Here's how the part is built. I have some questions about the finished solid (model axes, mm). Coordinates: 2 decimals unless noted, no trailing zeros. Write each loop counter-clockwise with the first axis right and the second up, starting at its lowest first coordinate (ties: lowest second). Pieces come first, ordered by that corner, then holes.
Item 1: I want a section at A-A (x = 0). Please give me the cut outline in (y, z), and give its area (3 significant figures).
Item 2: I want a section at D-D (z = 22). Please give me the cut outline in (x, y), and give its area (3 significant figures).
Item 3: I'm going to push flat-ended pins straight in: P1, Ø14.5, axis at x = 0, y = 0, coming from the -Z side; P2, Ø2, axis at y = -10, z = 10.5, coming from the -X side; P3, Ø1.5, axis at y = 42.5, z = 15, coming from the +X side; P4, Ø5, axis at x = -24, z = -6, coming from the +Y side. Where does each tip first touch, or does it pass through?
Item 4: Please list where these lines run through material, in increasing order: line 1 (Y direction, x = 0, z = 7.25); line 2 (Y direction, x = 0, z = -15).
Item 5: I want a section at C-C (z = -4). Please give me the cut outline in (x, y), and give its area (3 significant figures).
from build123d import *

# Parameters (mm, degrees)
SKETCH2_R               = 6.35
CUT_EXTRUDE1_DEPTH      = 108.458
CUT_EXTRUDE1_DEPTH_BACK = 134.62


with BuildPart() as part:
    # Sketch1 → Revolve2 (revolve)
    with BuildSketch(Plane(origin=(0, 0, 0), x_dir=(0, 0, -1), z_dir=(1, 0, 0))):
        with BuildLine():
            Line((-25.4, 0), (-25.4, 58.42))
            ThreePointArc((-25.4, 58.42), (-20.192358569, 70.992358569), (-7.62, 76.2))
            Line((-7.62, 76.2), (7.62, 76.2))
            ThreePointArc((7.62, 76.2), (20.192358569, 70.992358569), (25.4, 58.42))
            Line((25.4, 58.42), (25.4, 0))
            Line((25.4, 0), (-25.4, 0))
        make_face()
    revolve(axis=Axis((0, 0, -37.220072608), (0, 0, 1)))

    # Sketch2 → Cut-Extrude1 (cut, two sides)
    with BuildSketch(Plane.XY) as cut_extrude1_sk:
        Circle(SKETCH2_R)
    extrude(amount=CUT_EXTRUDE1_DEPTH, mode=Mode.SUBTRACT)
    extrude(cut_extrude1_sk.sketch, amount=-CUT_EXTRUDE1_DEPTH_BACK, mode=Mode.SUBTRACT)


solid = part.part
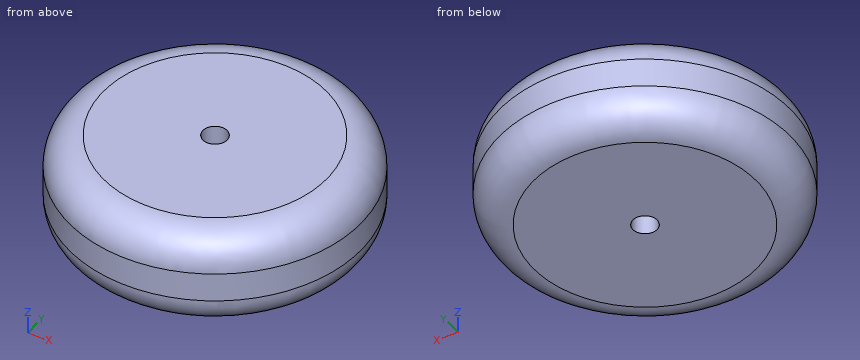
Answer:
1. outline: (-76.2, -7.62) arc R17.78 ccw to (-58.42, -25.4) - (-6.35, -25.4) - (-6.35, 25.4) - (-58.42, 25.4) arc R17.78 ccw to (-76.2, 7.62) - close; (6.35, -25.4) - (58.42, -25.4) arc R17.78 ccw to (76.2, -7.62) - (76.2, 7.62) arc R17.78 ccw to (58.42, 25.4) - (6.35, 25.4) - close
1. area: 6,830 mm2
2. outline: circle Ø137.75 at (0, 0); hole circle Ø12.7 at (0, 0)
2. area: 14,800 mm2
3. P1: stops at z = -25.4
3. P2: stops at x = -75.5
3. P3: stops at x = 61.96
3. P4: stops at y = 73.1
4. line 1: y = -76.2 to -6.35, 6.35 to 76.2
4. line 2: y = -74.6 to -6.35, 6.35 to 74.6
5. outline: circle Ø152.4 at (0, 0); hole circle Ø12.7 at (0, 0)
5. area: 18,100 mm2
